```python
from build123d import *

# Parameters (mm, degrees)
F1_DEPTH  = 203.454
F2_T      = -2.54
F3_W      = 139.7
F3_H      = 6.35
F4_DEPTH  = 6.35
F5_W      = 139.7
F5_H      = 6.35
F6_DEPTH  = 6.35
F7_W      = 185.674
F7_H      = 6.35
F8_DEPTH  = 6.35
F10_DEPTH = 203.455
F12_DEPTH = 203.455


with BuildPart() as f1:
    # F0 (on Right) → F1 (new body)
    with BuildSketch(Plane.YZ):
        Polygon((-107.919275, 0), (95.280725, 0), (95.280725, 50.8), align=None)
    extrude(amount=F1_DEPTH)

    # F2
    f2_openings = [f1.faces().sort_by_distance(p)[0] for p in [
        (101.727, -6.319275, 0),
    ]]
    offset(amount=F2_T, openings=f2_openings)

    # F3 (on face) → F4 (join)
    with BuildSketch(Plane.YZ.offset(2.54)):
        with Locations((22.890725, 6.35)):
            Rectangle(F3_W, F3_H)
    extrude(amount=F4_DEPTH)

    # F5 (on face) → F6 (join)
    with BuildSketch(Plane(origin=(200.914, 0, 0), x_dir=(0, -1, 0), z_dir=(-1, 0, 0))):
        with Locations((-22.890725, 6.35)):
            Rectangle(F5_W, F5_H)
    extrude(amount=F6_DEPTH)

    # F7 (on face) → F8 (join)
    with BuildSketch(Plane.XZ.offset(-92.740725)):
        with Locations((101.727, 6.35)):
            Rectangle(F7_W, F7_H)
    extrude(amount=F8_DEPTH)

    # F9 (on face) → F10 (cut, through all)
    with BuildSketch(Plane.YZ.offset(203.454)):
        with BuildLine():
            Line((78.135725, 0), (84.485725, 0))
            Line((84.485725, 0), (84.485725, 23.8125))
            ThreePointArc((84.485725, 23.8125), (84.020757, 24.935032), (82.898225, 25.4))
            Line((82.898225, 25.4), (79.723225, 25.4))
            ThreePointArc((79.723225, 25.4), (78.600693, 24.935032), (78.135725, 23.8125))
            Line((78.135725, 23.8125), (78.135725, 0))
        make_face()
    extrude(amount=-F10_DEPTH, mode=Mode.SUBTRACT)

    # F11 (on face) → F12 (cut, through all)
    with BuildSketch(Plane(origin=(0, 0, 0), x_dir=(0, -1, 0), z_dir=(-1, 0, 0))):
        with BuildLine():
            ThreePointArc((0.128145, 13.311182), (2.521184, 10.95378), (4.890525, 13.335))
            ThreePointArc((4.890525, 13.335), (2.497366, 15.71622), (0.128145, 13.311182))
        make_face()
        with BuildLine():
            Line((4.890525, 0), (4.890525, 13.335))
            ThreePointArc((4.890525, 13.335), (2.521184, 10.95378), (0.128145, 13.311182))
            Line((0.128145, 13.311182), (0.128145, 0))
            Line((0.128145, 0), (4.890525, 0))
        make_face()
    extrude(amount=-F12_DEPTH, mode=Mode.SUBTRACT)


solid = f1.part
```
Can you work these out from the model? Positions are in its coordinate system, mm. A direction names the side the tool comes from. Give positions to 0.01 mm unless a question says otherwise; leave off trailing zeros. Loops run counter-clockwise (first coordinate to the right, second up) from the corner with the lowest first, then second, coordinate; pieces in that order, holes last. Notation, with made-up numbers: M 71.25,67 L 114.25,67 A15 ccw 114.25,87 Z; hole C 56,-11.5 d4. An arc over 180 degrees is marked long. Use CSV: the item, a comma, the result in double quotes. Start each with the question number.
1. If we mould it in two halves opening along X, with no side actions, what happens to faces 1 (the face through (4, 84.486, 9)), 2 (the face through (198, -46.959, 6))? For each: released by +X, released by -X, zero draft, split by the parting line, or undercut.
2. For P1, Ø3.5, axis at y = 90, z = 1.5, coming from the -X side; P2, Ø5, axis at x = 196.5, y = -17, coming from the +Z side; P3, Ø5, axis at x = 199, y = 58.5, coming from the +Z side; P4, Ø1, axis at x = 86.5, y = -26.5, coming from the +Z side, each with a flat end and sliding along its axis, tell me the tip position at first contact or that it passes through.
3. On a 3-axis mill with a long thin cutter (end or side, diameter ignored), from which of +Z, -Z, +X, -X, +Y, -Y can I reach the whole of each face in a straight line? I mean faces 3 (the face through (6, -26, 9.525)), 4 (the face through (101, -102, 0)), 5 (the face through (6, 40, 3.175)), 6 (the face through (200, -4.891, 7)). Say none if no direction works.
4. If I drill on L1, parallel to X at y = 27, z = 16.5; L2, parallel to Z at x = 40, y = 12; L3, parallel to Z at x = 43, y = 40, over which ranges is the centre line in solid material (lowest first)?
5. Imagine slicing it at A-A, the plane z = 45. Write out the boundary of the cut face in (x, y).
6. Imagine slicing it at B-B, the plane x = 68. Write out the boundary of the cut face in (y, z) (3 decimals), plus the area to 3 significant figures.
7. Imagine slicing it at C-C, the plane y = 67.5. Write out the boundary of the cut face in (x, z) (3 decimals).
8. Imagine slicing it at D-D, the plane z = 29. Write out the boundary of the cut face in (x, y).
Response values:
1,face 1,"zero draft"
1,face 2,"undercut"
2,P1,"x = 0"
2,P2,"z = 23.35"
2,P3,"z = 42.23"
2,P4,"z = 20.48"
3,face 3,"none"
3,face 4,"-Z, +X, -X, +Y, -Y"
3,face 5,"-Z"
3,face 6,"-Z, +X, -X"
4,L1,"0 to 2.54, 200.91 to 203.45"
4,L2,"27.36 to 29.98"
4,L3,"34.36 to 36.98"
5,outline,"M 0,72.08 L 203.45,72.08 L 203.45,95.28 L 0,95.28 Z; hole M 2.54,82.55 L 200.91,82.55 L 200.91,92.74 L 2.54,92.74 Z"
6,outline,"M -107.919,0 L -97.447,0 L 92.741,47.547 L 92.741,9.525 L 86.391,9.525 L 86.391,3.175 L 92.741,3.175 L 92.741,0 L 95.281,0 L 95.281,50.8 Z"
6,area,"680 mm^2"
7,outline,"M 0,0 L 2.54,0 L 2.54,3.175 L 8.89,3.175 L 8.89,9.525 L 2.54,9.525 L 2.54,41.237 L 200.914,41.237 L 200.914,9.525 L 194.564,9.525 L 194.564,3.175 L 200.914,3.175 L 200.914,0 L 203.454,0 L 203.454,43.855 L 0,43.855 Z"
8,outline,"M 0,8.08 L 203.45,8.08 L 203.45,95.28 L 0,95.28 Z; hole M 2.54,18.55 L 200.91,18.55 L 200.91,92.74 L 2.54,92.74 Z"
